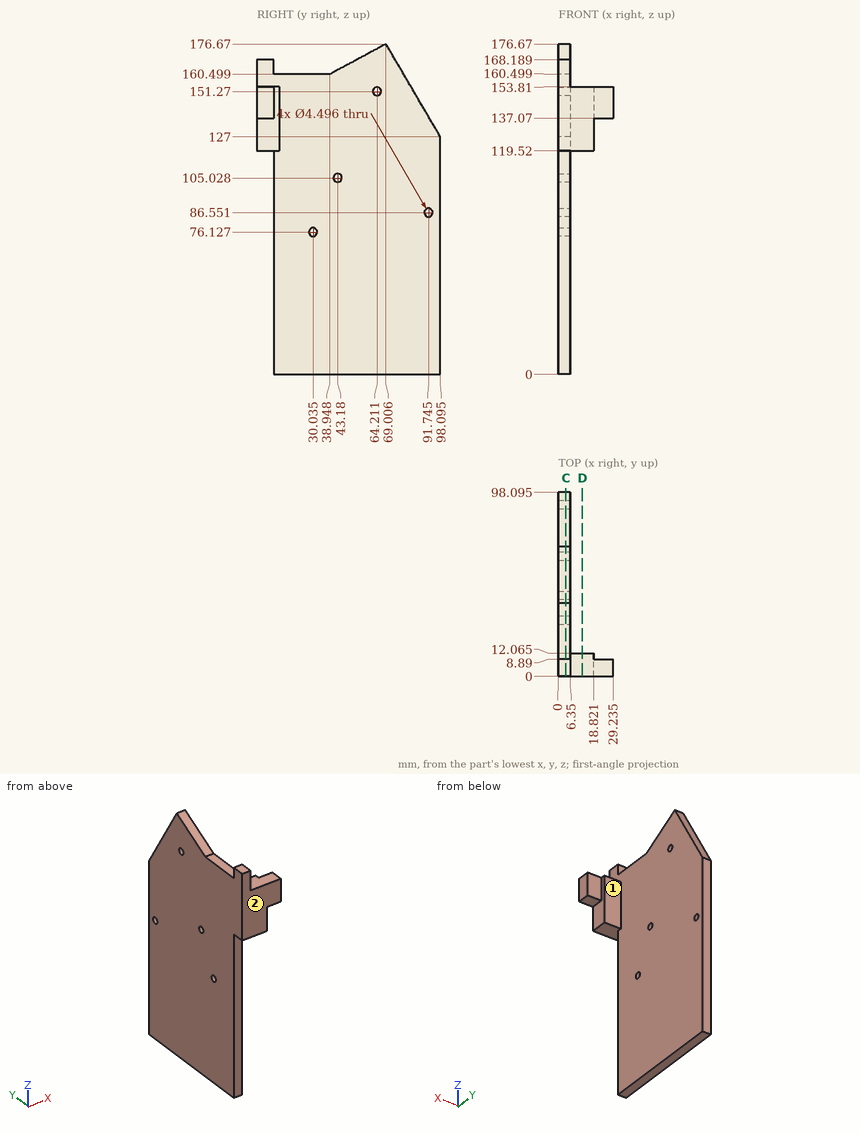
Part print with two shaded views. Sizes in mm from the minimum x, y, z corner. A direction names the side the tool comes from. Round coordinates to 2 decimals unless told otherwise and drop trailing zeros. Loops run counter-clockwise (first coordinate to the right, second up) from the corner with the lowest first, then second, coordinate; pieces in that order, holes last. Notation, with made-up numbers: M -20.75,-5.5 L 27.25,-5.5 A14 cw 27.25,13.5 Z; hole C -27,76.5 d9. An arc over 180 degrees is marked long. Put each result on its own line as item: value. Start each with the question number.
Item 1: 3-axis set-ups, long thin cutter, end or side, ignore diameter. For the marked faces 1 and 2: which of +Z, -Z, +X, -X, +Y, -Y reach the whole face in a straight line?
Item 2: Drill centre lines: line 1 along X through (y, z) = (26.5, 23.5); line 2 along X through (y, z) = (6, 125); line 3 along Z through (x, y) = (5.75, 27). Where is each one in solid material? Low to high.
Item 3: Cut at D-D (x = 12.75). List the corners of the cut face in (y, z) (1 decimal).
Item 4: Drop flat-ended pins along their axis: P1, Ø2.5, axis at x = 25, y = 4.5, coming from the -Z side; P2, Ø5, axis at x = 6, y = 40.5, coming from the +Z side; P3, Ø4, axis at x = 17, z = 118.5, coming from the +Y side (1 decimal). Give the stop position or say it passes through.
Item 5: Cut at C-C (x = 4). Give the number of separate pieces and of enclosed holes in the cut face, then the cut area to 3 significant figures.
Answer block:
1. face 1: +Z, -Z, +X, +Y
1. face 2: +Z, -Z, +X, -X, -Y
2. line 1: 0 to 6.35
2. line 2: 0 to 18.82
2. line 3: 0 to 160.5
3. outline: M 0,119.5 L 12.1,119.5 L 12.1,153.8 L 0,153.8 Z
4. P1: z = 137.07
4. P2: z = 162.68
4. P3: y = 12.1
5. separate pieces: 1
5. enclosed holes: 4
5. area: 14,700 mm2
